Read the model definition and answer for the solid it produces. Units are mm, in the model's axes. Give positions to 0.01 mm unless a question says otherwise; leave off trailing zeros. Order: outer loops, then holes, each group sorted by start corner. A loop starts at its lowest first (then second) coordinate and runs counter-clockwise, first axis right, second up.
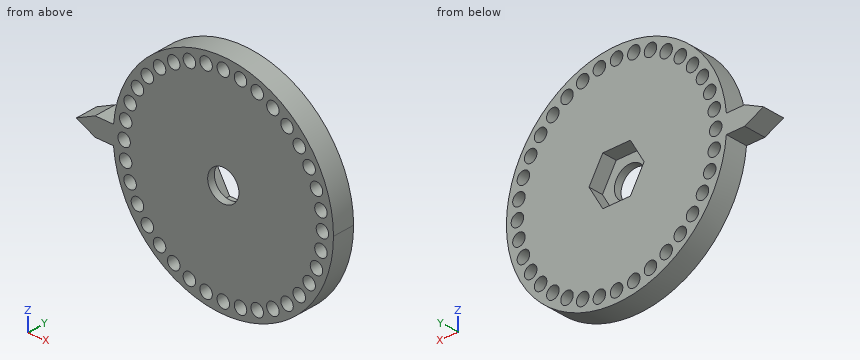
```python
from build123d import *

# Parameters (mm, degrees)
SKETCH1_R           = 30
BOSS_EXTRUDE1_DEPTH = 6
CUT_EXTRUDE1_DEPTH  = 4
SKETCH3_R           = 1.7
CUT_EXTRUDE2_DEPTH  = 7
CIRPATTERN1_COUNT   = 36
SKETCH4_R           = 4.25
CUT_EXTRUDE3_DEPTH  = 3
BOSS_EXTRUDE2_DEPTH = 6


with BuildPart() as part:
    # Sketch1 → Boss-Extrude1 (new body)
    with BuildSketch(Plane(origin=(0, 0, 0), x_dir=(1, 0, 0), z_dir=(0, 1, 0))):
        Circle(SKETCH1_R)
    extrude(amount=BOSS_EXTRUDE1_DEPTH)

    # Sketch2 → Cut-Extrude1 (cut)
    with BuildSketch(Plane(origin=(0, 6, 0), x_dir=(1, 0, 0), z_dir=(0, 1, 0))):
        Polygon((3.75277675, 6.5), (-3.75277675, 6.5), (-7.505553499, 0), (-3.75277675, -6.5), (3.75277675, -6.5), (7.505553499, 0), align=None)
    extrude(amount=-CUT_EXTRUDE1_DEPTH, mode=Mode.SUBTRACT)

    # Sketch3 → Cut-Extrude2 (cut, through all)
    with BuildSketch(Plane(origin=(0, 6, 0), x_dir=(1, 0, 0), z_dir=(0, 1, 0))):
        with Locations((0, 27)):
            Circle(SKETCH3_R)
    cut_extrude2 = extrude(amount=-CUT_EXTRUDE2_DEPTH, mode=Mode.SUBTRACT)

    # CirPattern1: Cut-Extrude2 ×36 about axis
    cirpattern1_axis = Axis((0, 0, 0), (0, 1, 0))
    for i in range(1, CIRPATTERN1_COUNT):
        add(cut_extrude2.rotate(cirpattern1_axis, i * 360 / CIRPATTERN1_COUNT), mode=Mode.SUBTRACT)

    # Sketch4 → Cut-Extrude3 (cut, through all)
    with BuildSketch(Plane(origin=(0, 2, 0), x_dir=(1, 0, 0), z_dir=(0, 1, 0))):
        Circle(SKETCH4_R)
    extrude(amount=-CUT_EXTRUDE3_DEPTH, mode=Mode.SUBTRACT)

    # Sketch5 → Boss-Extrude2 (add)
    with BuildSketch(Plane(origin=(0, 6, 0), x_dir=(1, 0, 0), z_dir=(0, 1, 0))):
        Polygon((-34.895651858, 2.5), (-40, 0), (-34.895651858, -2.5), (-29.895651858, -2.5), (-29.895651858, 2.5), align=None)
    extrude(amount=-BOSS_EXTRUDE2_DEPTH)


solid = part.part
```
1) The part is cut by section C-C on x = 13.5. Determine the outline of the cut face in (y, z).
Final values:
outline: (0, -26.79) - (6, -26.79) - (6, -25.08) - (0, -25.08) - close; (0, -21.68) - (6, -21.68) - (6, 21.68) - (0, 21.68) - close; (0, 25.08) - (6, 25.08) - (6, 26.79) - (0, 26.79) - close
2) The part is cut by section D-D on y = 4.15. Count the separate pieces of the cut face and the enclosed holes in it, and give its area (3 significant figures).
Final values:
separate pieces: 1
enclosed holes: 37
area: 2,390 mm2
3) Given pin 1 (1.5 mm diameter, centred on x = -31, y = 1, fed in from +Z); pin 2 (2.5 mm diameter, centred on x = 27, z = 0, fed in from -Y); pin 3 (1.5 mm diameter, centred on x = -32, y = 1.5, fed in from -Z); pin 4 (1.5 mm diameter, centred on y = 5, z = -13, fed in from -X) (3 decimals), each flat-ended and moving along its own axis, determine where each tip first touches the part or whether it passes through.
Final values:
pin 1: stops at z = 2.5
pin 2: passes through
pin 3: stops at z = -2.5
pin 4: stops at x = -27.385
4) The part is cut by section A-A on x = 0. Determine the outline of the cut face in (y, z), and give its area (3 significant figures).
Final values:
outline: (0, -30) - (6, -30) - (6, -28.7) - (0, -28.7) - close; (0, -25.3) - (6, -25.3) - (6, -6.5) - (2, -6.5) - (2, -4.25) - (0, -4.25) - close; (0, 4.25) - (2, 4.25) - (2, 6.5) - (6, 6.5) - (6, 25.3) - (0, 25.3) - close; (0, 28.7) - (6, 28.7) - (6, 30) - (0, 30) - close
area: 250 mm2
5) The part is cut by section B-B on z = 13.5. Determine the outline of the cut face in (x, y).
Final values:
outline: (-26.79, 0) - (-25.08, 0) - (-25.08, 6) - (-26.79, 6) - close; (-21.68, 0) - (21.68, 0) - (21.68, 6) - (-21.68, 6) - close; (25.08, 0) - (26.79, 0) - (26.79, 6) - (25.08, 6) - close
6) Consider L1, parallel to Z at x = 8, y = 1.65; L2, parallel to Z at x = -14.5, y = 3; L3, parallel to X at y = 1.7, z = 5.5. Determine where each line is inside the solid, lowest interval first.
Final values:
L1: z = -28.91 to -26.54, -24.2 to 24.2, 26.54 to 28.91
L2: z = -26.26 to -24.76, -22.01 to 22.01, 24.76 to 26.26
L3: x = -29.49 to -28.08, -25.1 to 25.1, 28.08 to 29.49
